Autodesk Inventor part; units mm, degrees
ref_plane "YZ Plane" through (0, 0, 0) normal (1, 0, 0) x (0, 1, 0)
ref_plane "XZ Plane" through (0, 0, 0) normal (0, 1, 0) x (-1, 0, 0)
ref_plane "XY Plane" through (0, 0, 0) normal (0, 0, 1) x (1, 0, 0)
sketch "Náčrt1" plane through (0, 0, 0) normal (1, 0, 0) x (0, 1, 0)
  line L0 (0, 0) -> (50, 0)
  line L1 (50, 0) -> (50, -50)
  line L2 (50, -50) -> (0, -50)
  line L3 (0, -50) -> (0, 0)
  arc A0 (0, -50) -> (50, 0) centre (0, 0) ccw
  line L4 (0, 0) -> (6, 0)
  line L5 (0, -6) -> (0, 0)
  line L6 (6, -6) -> (26, -6)
  line L7 (26, -6) -> (26, -26)
  line L8 (26, -26) -> (6, -26)
  line L9 (6, -26) -> (6, -6)
  dimension "d0" = 50
  dimension "d1" = 50
  dimension "d2" = 50
  dimension "d4" = 6
  dimension "d5" = 6
  dimension "d6" = 20
  dimension "d7" = 20
extrude "Vysunutí1" add sketch "Náčrt1" against normal blind 50 contours L0 A0 L3 | L1 L2 A0 | L6 L7 L8 L9
revolve "Rotace1" cut sketch "Náčrt1" angle 90 about axis through (0, 0, 0) along (0, 1, 0) keep common part contours L0 A0 L3 | L6 L7 L8 L9
extrude "Vysunutí2" add sketch "Náčrt1" along normal blind 50 contours L6 L7 L8 L9
sketch "Náčrt2" plane through (0, 6, -6) normal (0, 0, 1) x (1, 0, 0)
  line L0 (50, 20) -> (50, 0)
  line L1 (0, 0) -> (50, 0)
  point P0 (0, -6)
  point P1 (30, 10)
  dimension "d13" = 20
  dimension "d21" = 10
hole "Díra1" at (30, 16, -6) direction (0, 0, -1) diameter 6 end through all countersink diameter 15 countersink angle 90
pattern_circular "Kruhové pole1" count 3 over 360 about axis through (0, 0, 0) along (-0.5774, 0.5774, -0.5774) of "Vysunutí2", "Díra1"
properties part number "ZakulacenaCast"
Build history of the part. All positions in model axes, mm. A direction names the side the tool comes from. Round coordinates to 2 decimals unless told otherwise and drop trailing zeros. Loops run counter-clockwise (first coordinate to the right, second up) from the corner with the lowest first, then second, coordinate; pieces in that order, holes last.
Item 1: Saw through at C-C (z = -16). List the corners of the cut face in (x, y), then the cut area to 3 significant figures.
Item 2: Saw through at D-D (y = 16). List the corners of the cut face in (x, z).
Item 3: Saw through at A-A (z = 30). List the corners of the cut face in (x, y), then the cut area to 3 significant figures.
Item 4: Drill centre lines: line 1 along X through (y, z) = (19.25, 30); line 2 along Y through (x, z) = (30, -21); line 3 along Y through (x, z) = (-23, 24). Where is each one in solid material? Low to high.
Item 5: Which spindle directions (+Z, -Z, +X, -X, +Y, -Y) get a long thin tool onto all of the face, cutting with end or side? Do faces 5 (the face through (-26, 16, 25)), 6 (the face through (25, 16, -26)), 7 (the face through (-16, 26, 25)). Say none if no direction does.
Item 6: Pin check, flat tips, straight feed: P1, Ø1.5, axis at x = -11, y = -29, coming from the +Z side; P2, Ø8, axis at y = -30, z = -16, coming from the +X side; P3, Ø6, axis at x = -13.5, z = 26, coming from the -Y side. Stop position of each tip, or through.
Item 7: Saw through at B-B (x = 30). List the corners of the cut face in (y, z).
Item 8: Two-plate mould, pull along Y, no slides. Class faces 1 (the face through (-16.71, 10.22, 26.8)), 2 (the face through (26.8, 16.71, -10.22)), 3 (the face through (-18, -30, -19)), 4 (the face through (-16, -25, -26)): released by +Y, released by -Y, zero draft, split by the parting line, or undercut.
Worked answers:
1. outline: (-47.37, 0) - (-26, 0) - (-26, -27) - (-10.5, -27) - (-6, -22.5) - (-6, 0) - (0, 0) - (0, 6) - (50, 6) - (50, 26) - (0, 26) - (0, 47.37) arc R47.37 ccw to start; (-26, -50) - (-6, -50) - (-6, -37.5) - (-10.5, -33) - (-26, -33) - close; hole circle Ø6 at (30, 16)
1. area: 3,590 mm2
2. outline: (-47.37, 0) arc R47.37 ccw to (0, -47.37) - (0, -26) - (27, -26) - (27, -10.5) - (22.5, -6) - (0, -6) - (0, 0) - (-6, 0) - (-6, 50) - (-26, 50) - (-26, 0) - close; (33, -26) - (50, -26) - (50, -6) - (37.5, -6) - (33, -10.5) - close; hole circle Ø6 at (-16, 30)
3. outline: (-26, 6) - (-23.5, 6) - (-19, 10.5) - (-19, 26) - (-26, 26) - close; (-13, 10.5) - (-8.5, 6) - (-6, 6) - (-6, 26) - (-13, 26) - close
3. area: 260 mm2
4. line 1: x = -26 to -19, -13 to -6
4. line 2: y = 6 to 13, 19 to 26
4. line 3: y = 6 to 26
5. face 5: +Z, -X, +Y, -Y
5. face 6: -Z, +X, +Y, -Y
5. face 7: +Z, +X, -X, +Y
6. P1: stops at z = -6
6. P2: stops at x = -9.5
6. P3: stops at y = 6
7. outline: (6, -26) - (13, -26) - (13, -10.5) - (8.5, -6) - (6, -6) - close; (19, -26) - (26, -26) - (26, -6) - (23.5, -6) - (19, -10.5) - close
8. face 1: released by -Y
8. face 2: undercut
8. face 3: undercut
8. face 4: zero draft
